Work out the finished part from the listing and answer in its coordinate system (mm). A direction names the side the tool comes from. Give positions to 0.01 mm unless a question says otherwise; leave off trailing zeros. Order: outer loops, then holes, each group sorted by start corner. A loop starts at its lowest first (then second) coordinate and runs counter-clockwise, first axis right, second up.
```python
from build123d import *

# Parameters (mm, degrees)
SKETCH1_R               = 31.75
BOSS_EXTRUDE1_DEPTH     = 19.05
CUT_EXTRUDE1_DEPTH      = 5.08
SKETCH4_R               = 0.539725026
CUT_EXTRUDE2_DEPTH      = 9.62045401
CUT_EXTRUDE2_DEPTH_BACK = 1.524


with BuildPart() as part:
    # Sketch1 → Boss-Extrude1 (new body)
    with BuildSketch(Plane(origin=(0, 0, 0), x_dir=(1, 0, 0), z_dir=(0, 1, 0))):
        Circle(SKETCH1_R)
    extrude(amount=BOSS_EXTRUDE1_DEPTH)

    # Sketch2 → Cut-Extrude1 (cut)
    with BuildSketch(Plane(origin=(0, 19.05, 0), x_dir=(1, 0, 0), z_dir=(0, 1, 0))):
        with BuildLine():
            Line((0.431861346, 25.396328392), (0.481566937, 29.206030084))
            ThreePointArc((0.481566937, 29.206030084), (-2.110193645, 29.133677811), (-4.685328245, 28.831784531))
            Line((-4.685328245, 28.831784531), (-4.021364533, 25.079645677))
            ThreePointArc((-4.021364533, 25.079645677), (-1.801722861, 25.336017736), (0.431861346, 25.396328392))
        make_face()
    extrude(amount=-CUT_EXTRUDE1_DEPTH, mode=Mode.SUBTRACT)

    # Sketch4 → Cut-Extrude2 (cut, two sides)
    with BuildSketch(Plane(origin=(-1.794751593, 0, -25.237987034), x_dir=(-0.997481013, 0, 0.070933971), z_dir=(-0.070933971, 0, -0.997481013))) as cut_extrude2_sk:
        with Locations((1.415895648, 18.077123557)):
            Circle(SKETCH4_R)
    extrude(amount=CUT_EXTRUDE2_DEPTH, mode=Mode.SUBTRACT)
    extrude(cut_extrude2_sk.sketch, amount=-CUT_EXTRUDE2_DEPTH_BACK, mode=Mode.SUBTRACT)


solid = part.part
```
1. The part is cut by section C-C (y = 4.75). Write down the section's boundary in (x, z).
Findings below:
outline: circle Ø63.5 at (0, 0)
2. The mould has two halves that part along Z. Classify faces 1 (the face through (-6.883, 9.392, 30.995)), 2 (the face through (0, 0, 0)), 3 (the face through (-2.074, 16.546, -29.136)): pulls with the +Z half, pulls with the -Z half, needs draft (parallel to the pull), parting line crosses it, or undercut.
Findings below:
face 1: parting line crosses it
face 2: needs draft
face 3: undercut
3. Given P1, Ø8, axis at x = -12.5, y = 5, coming from the -Z side; P2, Ø1.5, axis at y = 11, z = -12.5, coming from the -X side; P3, Ø10, axis at y = 16, z = 7.5, coming from the +X side, each flat-ended and moving along its own axis, determine where each tip first touches the part or whether it passes through.
Findings below:
P1: stops at z = -30.59
P2: stops at x = -29.5
P3: stops at x = 31.65
4. The part is cut by section D-D (x = -8). Write down the section's boundary in (y, z).
Findings below:
outline: (0, -30.73) - (19.05, -30.73) - (19.05, 30.73) - (0, 30.73) - close
5. Straight lines are drawn through the part: probe 1 along X at (y, z) = (6.75, 13); probe 2 along Z at (x, y) = (23.5, 5.25); probe 3 along Z at (x, y) = (-27, 16.25). For each, find the intervals that lie inside material, in ascending order.
Findings below:
probe 1: x = -28.97 to 28.97
probe 2: z = -21.35 to 21.35
probe 3: z = -16.71 to 16.71
6. The part is cut by section A-A (y = 15). Write down the section's boundary in (x, z), then the cut area to 3 significant figures.
Findings below:
outline: circle Ø63.5 at (0, 0); hole (-4.69, -28.83) arc R29.21 ccw to (0.48, -29.21) - (0.43, -25.4) arc R25.4 cw to (-4.02, -25.08) - close
area: 3,150 mm2
7. Which of the six approach directions +Z, -Z, +X, -X, +Y, -Y give full straight-line access (tool end or side, diameter ignored) to faces 4 (the face through (0, 19.05, 0)), 5 (the face through (-2, 13.97, -27))?
Findings below:
face 4: +Z, -Z, +X, -X, +Y
face 5: +Y
8. The part is cut by section B-B (z = 20). Write down the section's boundary in (x, y).
Findings below:
outline: (-24.66, 0) - (24.66, 0) - (24.66, 19.05) - (-24.66, 19.05) - close
